```python
from build123d import *

# Parameters (mm, degrees)
BOSS_EXTRUDE1_DEPTH                              = 44.45
CBORE_FOR_1_4_SOCKET_SHOULDER_SCREW1_D           = 6.5278
CBORE_FOR_1_4_SOCKET_SHOULDER_SCREW1_CBORE_D     = 10.31748
CBORE_FOR_1_4_SOCKET_SHOULDER_SCREW1_CBORE_DEPTH = 3.302


with BuildPart() as part:
    # Sketch1 → Boss-Extrude1 (new body)
    with BuildSketch(Plane(origin=(0, 0, 0), x_dir=(0, 0, -1), z_dir=(1, 0, 0))):
        Polygon((-25.4, 31.75), (-19.05, 31.75), (-19.05, 6.35), (0, 6.35), (0, 0), (-25.4, 0), align=None)
    extrude(amount=BOSS_EXTRUDE1_DEPTH)

    # CBORE for 1/4 Socket Shoulder Screw1 (through all)
    with Locations(Plane(origin=(0, 6.35, 0), x_dir=(1, 0, 0), z_dir=(0, 1, 0))):
        with Locations((9.525, -6.985), (34.925, -6.985)):
            CounterBoreHole(CBORE_FOR_1_4_SOCKET_SHOULDER_SCREW1_D / 2, CBORE_FOR_1_4_SOCKET_SHOULDER_SCREW1_CBORE_D / 2, CBORE_FOR_1_4_SOCKET_SHOULDER_SCREW1_CBORE_DEPTH)


solid = part.part
```
Build history of the part. All positions in model axes, mm. A direction names the side the tool comes from. Give positions to 0.01 mm unless a question says otherwise; leave off trailing zeros. Loops run counter-clockwise (first coordinate to the right, second up) from the corner with the lowest first, then second, coordinate; pieces in that order, holes last.
1) Two-plate mould, pull along X, no slides. Class faces 4 (the face through (4.37, 4.72, 6.76)), 5 (the face through (0, 9, 21)), 6 (the face through (22, 6.35, 10)): released by +X, released by -X, zero draft, split by the parting line, or undercut.
Values follow:
face 4: undercut
face 5: released by -X
face 6: zero draft
2) Band-saw the part on C-C on x = 41.5. List the corners of the cut face in (y, z).
Values follow:
outline: (0, 0) - (6.35, 0) - (6.35, 19.05) - (31.75, 19.05) - (31.75, 25.4) - (0, 25.4) - close
3) Probe line 1 along X through (y, z) = (1, 5.75); line 2 along X through (y, z) = (3.5, 3.5); line 3 along Y through (x, z) = (18.5, 16). List the from-to ranges inside material, lowest first.
Values follow:
line 1: x = 0 to 6.5, 12.55 to 31.9, 37.95 to 44.45
line 2: x = 0 to 5.72, 13.33 to 31.12, 38.73 to 44.45
line 3: y = 0 to 6.35
4) Band-saw the part on A-A on z = 4.25. List the corners of the cut face in (x, y).
Values follow:
outline: (0, 0) - (7.74, 0) - (7.74, 3.05) - (5.15, 3.05) - (5.15, 6.35) - (0, 6.35) - close; (11.31, 0) - (33.14, 0) - (33.14, 3.05) - (30.55, 3.05) - (30.55, 6.35) - (13.9, 6.35) - (13.9, 3.05) - (11.31, 3.05) - close; (36.71, 0) - (44.45, 0) - (44.45, 6.35) - (39.3, 6.35) - (39.3, 3.05) - (36.71, 3.05) - close
5) Band-saw the part on B-B on x = 33.5. List the corners of the cut face in (y, z).
Values follow:
outline: (0, 0) - (6.35, 0) - (6.35, 2.03) - (3.05, 2.03) - (3.05, 4.05) - (0, 4.05) - close; (0, 9.92) - (3.05, 9.92) - (3.05, 11.94) - (6.35, 11.94) - (6.35, 19.05) - (31.75, 19.05) - (31.75, 25.4) - (0, 25.4) - close
6) Drop flat-ended pins along their axis: P1, Ø5.5, axis at x = 14.5, z = 11, coming from the +Y side; P2, Ø7.5, axis at x = 30.5, y = 20, coming from the -Z side; P3, Ø7.5, axis at x = 9.525, z = 6.985, coming from the +Y side. Give the stop position or say it passes through.
Values follow:
P1: stops at y = 6.35
P2: stops at z = 19.05
P3: stops at y = 3.05
7) Band-saw the part on D-D on y = 5. List the corners of the cut face in (x, z) (3 decimals), then the cut area to 3 significant figures.
Values follow:
outline: (0, 0) - (44.45, 0) - (44.45, 25.4) - (0, 25.4) - close; hole circle Ø10.317 at (9.525, 6.985); hole circle Ø10.317 at (34.925, 6.985)
area: 962 mm2
8) 3-axis set-ups, long thin cutter, end or side, ignore diameter. For faces 1 (the face through (9.5, 3.048, 10.4)), 2 (the face through (6.412, 1.503, 6.005)), 3 (the face through (22, 19, 19.05)): which of +Z, -Z, +X, -X, +Y, -Y reach the whole face in a straight line?
Values follow:
face 1: +Y
face 2: +Y, -Y
face 3: -Z, +X, -X, +Y
